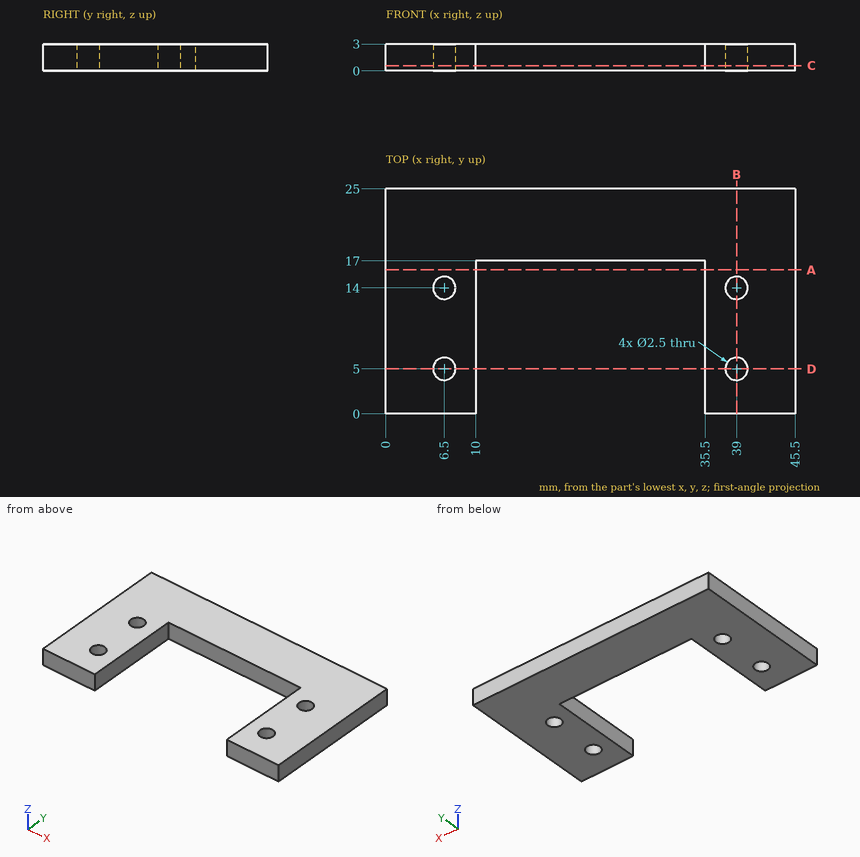
Geometry: see drawing. Coordinates: mm, zero at the bounding-box minimum. Give positions to 0.01 mm unless a question says otherwise; leave off trailing zeros. Loops run counter-clockwise (first coordinate to the right, second up) from the corner with the lowest first, then second, coordinate; pieces in that order, holes last. Notation, with made-up numbers: (87.5, 76.5) -> (109.5, 76.5) arc R26 cw to (109.5, 106.5) -> close; hole circle Ø3 at (87.5, 66.25). An arc over 180 degrees is marked (long way). Answer as a JSON object with one key per item and string values. Group by question number.
Item 1: Pin query (flat end, axial travel): P1, Ø1.5, axis at x = 21.5, z = 2, coming from the -Y side. Return the tip coordinate at first contact, or that it passes through.
Item 2: Cut plane D-D, the plane y = 5. Return the cut outline in (x, z), and give its area (3 significant figures).
Item 3: Cut plane A-A, the plane y = 16. Return the cut outline in (x, z), and give its area (3 significant figures).
Item 4: Cut plane B-B, the plane x = 39. Return the cut outline in (y, z), and give its area (3 significant figures).
Item 5: Line query: probe 1 along Y at (x, z) = (6.5, 2.05); probe 2 along X at (y, z) = (6.75, 1.15); probe 3 along Y at (x, z) = (6, 0.35). Output: solid intervals per line, ascending.
Item 6: Cut plane C-C, the plane z = 0.6. Return the cut outline in (x, y), and give its area (3 significant figures).
Checks:
{
 "1": {"P1": "stops at y = 17"},
 "2": {"outline": "(0, 0) -> (5.25, 0) -> (5.25, 3) -> (0, 3) -> close; (7.75, 0) -> (10, 0) -> (10, 3) -> (7.75, 3) -> close; (35.5, 0) -> (37.75, 0) -> (37.75, 3) -> (35.5, 3) -> close; (40.25, 0) -> (45.5, 0) -> (45.5, 3) -> (40.25, 3) -> close", "area": "45.0 mm²"},
 "3": {"outline": "(0, 0) -> (10, 0) -> (10, 3) -> (0, 3) -> close; (35.5, 0) -> (45.5, 0) -> (45.5, 3) -> (35.5, 3) -> close", "area": "60.0 mm²"},
 "4": {"outline": "(0, 0) -> (3.75, 0) -> (3.75, 3) -> (0, 3) -> close; (6.25, 0) -> (12.75, 0) -> (12.75, 3) -> (6.25, 3) -> close; (15.25, 0) -> (25, 0) -> (25, 3) -> (15.25, 3) -> close", "area": "60.0 mm²"},
 "5": {"probe 1": "y = 0 to 3.75, 6.25 to 12.75, 15.25 to 25", "probe 2": "x = 0 to 10, 35.5 to 45.5", "probe 3": "y = 0 to 3.85, 6.15 to 12.85, 15.15 to 25"},
 "6": {"outline": "(0, 0) -> (10, 0) -> (10, 17) -> (35.5, 17) -> (35.5, 0) -> (45.5, 0) -> (45.5, 25) -> (0, 25) -> close; hole circle Ø2.5 at (6.5, 5); hole circle Ø2.5 at (6.5, 14); hole circle Ø2.5 at (39, 5); hole circle Ø2.5 at (39, 14)", "area": "684 mm²"}
}
